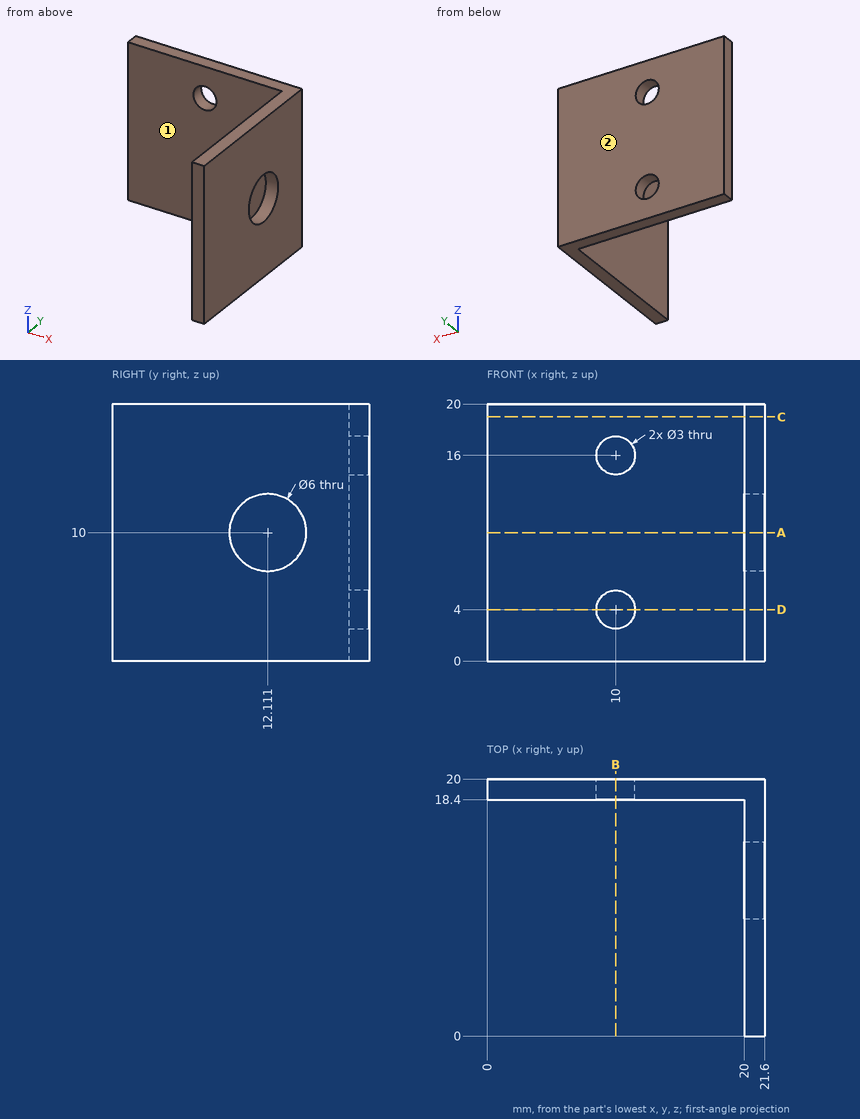
Source: three-view drawing plus pictorial views. Frame: mm from the lowest corner of the part. A direction names the side the tool comes from. Coordinates: 2 decimals unless noted, no trailing zeros. Write each loop counter-clockwise with the first axis right and the second up, starting at its lowest first coordinate (ties: lowest second). Pieces come first, ordered by that corner, then holes. Notation, with made-up numbers: (-32.75, -11.5) -> (-19.75, -11.5) arc R12 ccw to (-19.75, 7.5) -> close; hole circle Ø9 at (2, 2). An arc over 180 degrees is marked (long way). Answer as a JSON object with one key per item and string values.
1. Access query for the marked faces 1 and 2. Directions: +Z, -Z, +X, -X, +Y, -Y. A direction counts if a zero-diameter tool reaches every point of the face in a straight line with its end or side. Return the directions, or none.
Result set:
{"face 1": "+Z, -Z, -X, -Y", "face 2": "+Z, -Z, +X, -X, +Y"}
2. Section A-A on z = 10. Return the cut outline in (x, y).
Result set:
{"outline": "(0, 18.4) -> (20, 18.4) -> (20, 15.11) -> (21.6, 15.11) -> (21.6, 20) -> (0, 20) -> close; (20, 0) -> (21.6, 0) -> (21.6, 9.11) -> (20, 9.11) -> close"}
3. First-contact query: P1, Ø5.5, axis at y = 6.5, z = 14, coming from the -X side; P2, Ø1.5, axis at x = 12, z = 4, coming from the -Y side. Flat tips, straight axial feed; report the tip coordinate or a pass-through.
Result set:
{"P1": "stops at x = 20", "P2": "stops at y = 18.4"}
4. Section C-C on z = 19. Return the cut outline in (x, y).
Result set:
{"outline": "(0, 18.4) -> (20, 18.4) -> (20, 0) -> (21.6, 0) -> (21.6, 20) -> (0, 20) -> close"}
5. Section D-D on z = 4. Return the cut outline in (x, y).
Result set:
{"outline": "(0, 18.4) -> (8.5, 18.4) -> (8.5, 20) -> (0, 20) -> close; (11.5, 18.4) -> (20, 18.4) -> (20, 0) -> (21.6, 0) -> (21.6, 20) -> (11.5, 20) -> close"}
6. Material intervals for line 1 (X direction, y = 18.85, z = 4); line 2 (Y direction, x = 14, z = 7); line 3 (X direction, y = 5.5, z = 15.25), sorted ascending. Write a range as from..to.
Result set:
{"line 1": "x = 0..8.5, 11.5..21.6", "line 2": "y = 18.4..20", "line 3": "x = 20..21.6"}
7. Section B-B on x = 10. Return the cut outline in (y, z), then the cut area to 3 significant figures.
Result set:
{"outline": "(18.4, 0) -> (20, 0) -> (20, 2.5) -> (18.4, 2.5) -> close; (18.4, 5.5) -> (20, 5.5) -> (20, 14.5) -> (18.4, 14.5) -> close; (18.4, 17.5) -> (20, 17.5) -> (20, 20) -> (18.4, 20) -> close", "area": "22.4 mm2"}
